Autodesk Inventor part; units mm, degrees
ref_plane "YZ Plane" through (0, 0, 0) normal (1, 0, 0) x (0, 1, 0)
ref_plane "XZ Plane" through (0, 0, 0) normal (0, 1, 0) x (-1, 0, 0)
ref_plane "XY Plane" through (0, 0, 0) normal (0, 0, 1) x (1, 0, 0)
sketch "Sketch1" plane through (0, 0, 0) normal (0, 0, 1) x (1, 0, 0)
  line L0 (-203.2, 0) -> (203.2, 0)
  line L1 (-228.6, -279.4) -> (-228.6, -25.4)
  line L2 (228.6, -25.4) -> (228.6, -279.4)
  line L3 (295.4508, -374.8728) -> (618.2873, -492.3757)
  line L4 (635, -516.2439) -> (635, -600.0586)
  line L5 (609.6, -625.4586) -> (482.6, -625.4586)
  line L6 (482.6, -625.4586) -> (-228.6, -279.4)
  arc A0 (228.6, -279.4) -> (295.4508, -374.8728) centre (330.2, -279.4) ccw
  line L7 (-165.1, -190.5) -> (-38.1, -190.5) construction
  line L8 (-38.1, -190.5) -> (-38.1, -63.5) construction
  line L9 (-38.1, -63.5) -> (-165.1, -63.5) construction
  line L10 (-165.1, -63.5) -> (-165.1, -190.5) construction
  line L11 (-165.1, -190.5) -> (-38.1, -63.5) construction
  line L12 (-38.1, -190.5) -> (-165.1, -63.5) construction
  circle A1 centre (-165.1, -63.5) radius 9.525
  circle A2 centre (-38.1, -63.5) radius 9.525
  circle A3 centre (-38.1, -190.5) radius 9.525
  circle A4 centre (-165.1, -190.5) radius 9.525
  circle A5 centre (152.4, -63.5) radius 9.6564
  circle A6 centre (152.4, -190.5) radius 9.525
  arc A7 (635, -516.2439) -> (618.2873, -492.3757) centre (609.6, -516.2439) ccw
  arc A8 (609.6, -625.4586) -> (635, -600.0586) centre (609.6, -600.0586) ccw
  arc A9 (228.6, -25.4) -> (203.2, 0) centre (203.2, -25.4) ccw
  arc A10 (-203.2, 0) -> (-228.6, -25.4) centre (-203.2, -25.4) ccw
  point P0 (0, 0)
  point P1 (-228.6, 0)
  point P2 (228.6, 0)
  point P3 (0, 0)
  point P4 (635, -498.4586)
  point P5 (635, -625.4586)
  point P6 (-101.6, -127)
  point P7 (635, -558.1512)
  point P8 (546.1, -625.4586)
  dimension "d0" = 127
  dimension "d1" = 457.2
  dimension "d2" = 101.6
  dimension "d3" = 110
  dimension "d5" = 152.4
  dimension "d7" = 19.05
  dimension "d8" = 127
  dimension "d9" = 127
  dimension "d10" = 63.5
  dimension "d11" = 63.5
  dimension "d12" = 76.2
  dimension "d13" = 635
  dimension "d14" = 25.4
  dimension "d16" = 254
extrude "Plate1" add sketch "Sketch1" along normal blind 9.525
sketch "Sketch2" plane through (-234.379, -291.2766, -13.208) normal (-0.4375367, -0.8992006, 0) x (0.8992006, -0.4375367, 0)
  line L0 (790.9248, 0) -> (0, 0)
  line L1 (0, 0) -> (0, -24.892)
  line L2 (0, -24.892) -> (790.9248, -24.892)
  line L3 (790.9248, -24.892) -> (790.9248, 0)
edge flange "Flange1" height 38.1 angle 90 thickness 9.525 bend radius 13.208 thickness toward (-0.4375367, -0.8992006, 0) relief tear relief width 9.525 relief depth 4.7625 edges at (127, -452.4293, 0) wall of the first edge with corners at (476.821, -637.3352, -13.208) (-234.379, -291.2766, -13.208) (-234.379, -291.2766, -38.1) (476.821, -637.3352, -38.1)
bend "Bend1"
corner "Corner1"
equation "\"d15\" = Thickness"
equation "\"d19\" = BendReliefWidth"
equation "\"d20\" = BendReliefDepth"
equation "\"d21\" = MinimumRemnant"
equation "\"d22\" = TransitionRadius"
equation "\"d25\" = BendRadius"
equation "\"d26\" = CornerReliefSize"
equation "\"d27\" = GapSize"
equation "\"d28\" = JacobiRadiusSize"
equation "\"BendReliefWidth\" = Thickness"
equation "\"BendReliefDepth\" = 0.5 * Thickness"
equation "\"CornerReliefSize\" = 4 * Thickness"
equation "\"MinimumRemnant\" = 2 * Thickness"
equation "\"TransitionRadius\" = BendRadius"
equation "\"JacobiRadiusSize\" = Thickness"
equation "\"GapSize\" = Thickness"
properties part number "Model-2_Sheet-LH" material "SS304"
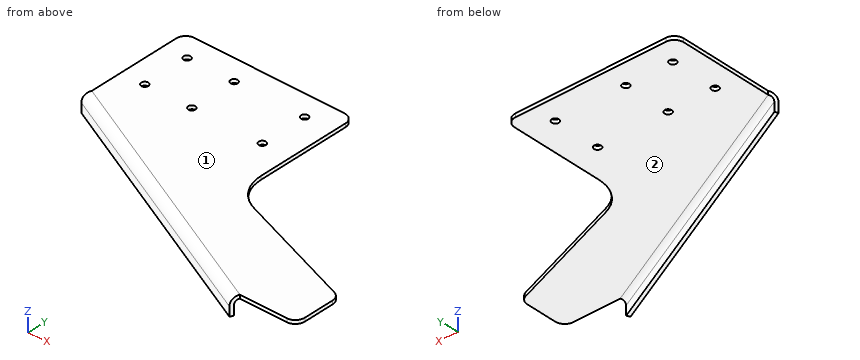
Design review of the part built by this model. Coordinates are the model's own, in mm. Face numbers are marked on the shaded views. A direction names the side the tool comes from. Round coordinates to 2 decimals unless told otherwise and drop trailing zeros. Write each loop counter-clockwise with the first axis right and the second up, starting at its lowest first coordinate (ties: lowest second). Pieces come first, ordered by that corner, then holes. Notation, with made-up numbers: (43.5, 59) - (58.5, 59) arc R10 ccw to (58.5, 65) - close; hole circle Ø11 at (63, -7.75). An arc over 180 degrees is marked (long way). Use a Markdown table: item, result. Add a question column.
1. We need section C-C (y = -190.5). State the section outline as (x, z) points (3 decimals).
2. We need section B-B (z = -20.5). State the section outline as (x, y) points.
3. Clearance check with flat-ended pins moving along their axes: pin 1 (10.5 mm diameter, centred on y = -183, z = 5, fed in from +X); pin 2 (2 mm diameter, centred on x = 185.5, z = -22, fed in from +Y); pin 3 (6 mm diameter, centred on y = -377.5, z = -27, fed in from -X); pin 4 (25 mm diameter, centred on x = -38.1, y = -63.5, fed in from +Z) (3 decimals). State where each tip first meets the part, or that it passes through.
4. We need section D-D (x = -165.1). Count the separate pieces of the cut face and the enclosed holes in it, then the cut area to 3 significant figures.
5. Wall thickness on probe 1 along Y at (x, z) = (-165.1, 4.5) (3 decimals); probe 2 along Y at (x, z) = (-165.1, 6.25) (3 decimals); probe 3 along Z at (x, y) = (-156, -26.5) (3 decimals): over which ranges is each line inside the solid? List them lowest first.
6. We need section A-A (y = -63.5). State the section outline as (x, z) points (3 decimals).
7. For the marked faces 1 and 2, list the 3-axis set-ups (+Z, -Z, +X, -X, +Y, -Y) from which the entire face can be reached by the end or side of a thin tool; tool diameter is ignored.
Output:
| question | item | result |
|---|---|---|
| 1 | outline | (-228.6, 0) - (-174.625, 0) - (-174.625, 9.525) - (-228.6, 9.525) - close; (-155.575, 0) - (-47.625, 0) - (-47.625, 9.525) - (-155.575, 9.525) - close; (-28.575, 0) - (142.875, 0) - (142.875, 9.525) - (-28.575, 9.525) - close; (161.925, 0) - (228.6, 0) - (228.6, 9.525) - (161.925, 9.525) - close |
| 2 | outline | (-238.55, -299.84) - (472.65, -645.9) - (476.82, -637.34) - (-234.38, -291.28) - close |
| 3 | pin 1 | stops at x = 228.6 |
| 3 | pin 2 | stops at y = -495.1 |
| 3 | pin 3 | stops at x = -85.11 |
| 3 | pin 4 | stops at z = 9.525 |
| 4 | separate pieces | 3 |
| 4 | enclosed holes | 0 |
| 4 | area | 3,160 mm2 |
| 5 | probe 1 | y = -326.151 to -200.025, -180.975 to -73.025, -53.975 to 0 |
| 5 | probe 2 | y = -323.371 to -200.025, -180.975 to -73.025, -53.975 to 0 |
| 5 | probe 3 | z = 0 to 9.525 |
| 6 | outline | (-228.6, 0) - (-174.625, 0) - (-174.625, 9.525) - (-228.6, 9.525) - close; (-155.575, 0) - (-47.625, 0) - (-47.625, 9.525) - (-155.575, 9.525) - close; (-28.575, 0) - (142.744, 0) - (142.744, 9.525) - (-28.575, 9.525) - close; (162.056, 0) - (228.6, 0) - (228.6, 9.525) - (162.056, 9.525) - close |
| 7 | face 1 | +Z, +X, -X, +Y, -Y |
| 7 | face 2 | -Z, +X, +Y |
